Autodesk Fusion 360 part; units mm, degrees
sketch "Sketch1" plane through (0, 0, 0) normal (0, 0, 1) x (1, 0, 0) in component "Washer"
  line L0 (100, -100) -> (-100, -100)
  line L1 (-100, -100) -> (-100, 100)
  line L2 (-100, 100) -> (100, 100)
  line L3 (100, 100) -> (100, -100)
  line L4 (100, -100) -> (-100, 100) construction
  line L5 (-100, -100) -> (100, 100) construction
  circle A0 centre (0, 0) radius 50
  dimension "d1" = 200
  dimension "d2" = 100
extrude "Extrude1" add sketch "Sketch1" along normal blind 20 in component "Washer"
component "Washer" placed x (1, 0, 0) y (0, 1, 0) z (0, 0, 1) at (0, 0, 0)
equation "d2 = d1 * 0.5"
The model under review builds one solid part; all positions refer to its coordinate system, in mm. Give positions to 0.01 mm unless a question says otherwise; leave off trailing zeros. Write each loop counter-clockwise with the first axis right and the second up, starting at its lowest first coordinate (ties: lowest second). Pieces come first, ordered by that corner, then holes.
(1) The part is to be moulded in two halves that separate along X. For faces 1 (the flat face through (-24, 46, 20)), 2 (the cylindrical face through (47.69, -15.02, 9.86)), 3 (the flat face through (100, 1, 10)), 4 (the flat face through (-100, -1, 10)), say which applies: released by +X, released by -X, zero draft, split by the parting line, or undercut.
(2) Consider section A-A, the plane x = 0. Give the boundary of the cut face in (y, z), and give its area (3 significant figures).
(3) Consider section C-C, the plane z = 11.25. Give the boundary of the cut face in (x, y), and give its area (3 significant figures).
(4) To check wall thickness, follow L1, parallel to Y at x = 0, z = 4.75; L2, parallel to X at y = 1, z = 4.5; L3, parallel to Y at x = 7, z = 7.5. State the ranges of each line that lie inside material, in increasing order.
Returned:
1. face 1: zero draft
1. face 2: undercut
1. face 3: released by +X
1. face 4: released by -X
2. outline: (-100, 0) - (-50, 0) - (-50, 20) - (-100, 20) - close; (50, 0) - (100, 0) - (100, 20) - (50, 20) - close
2. area: 2,000 mm2
3. outline: (-100, -100) - (100, -100) - (100, 100) - (-100, 100) - close; hole circle Ø100 at (0, 0)
3. area: 32,100 mm2
4. L1: y = -100 to -50, 50 to 100
4. L2: x = -100 to -49.99, 49.99 to 100
4. L3: y = -100 to -49.51, 49.51 to 100
